Geometry check sheet. Reference: drawing and pictorial views, mm from the part's lowest x, y, z. A direction names the side the tool comes from. Give positions to 0.01 mm unless a question says otherwise; leave off trailing zeros. Loops run counter-clockwise (first coordinate to the right, second up) from the corner with the lowest first, then second, coordinate; pieces in that order, holes last. Notation, with made-up numbers: (20.25, 16.25) -> (68.25, 16.25) arc R24 ccw to (68.25, 34.25) -> close; hole circle Ø1 at (11.5, 43.25). An arc over 180 degrees is marked (long way). Answer in a Markdown table with one row per item. Add a question column.
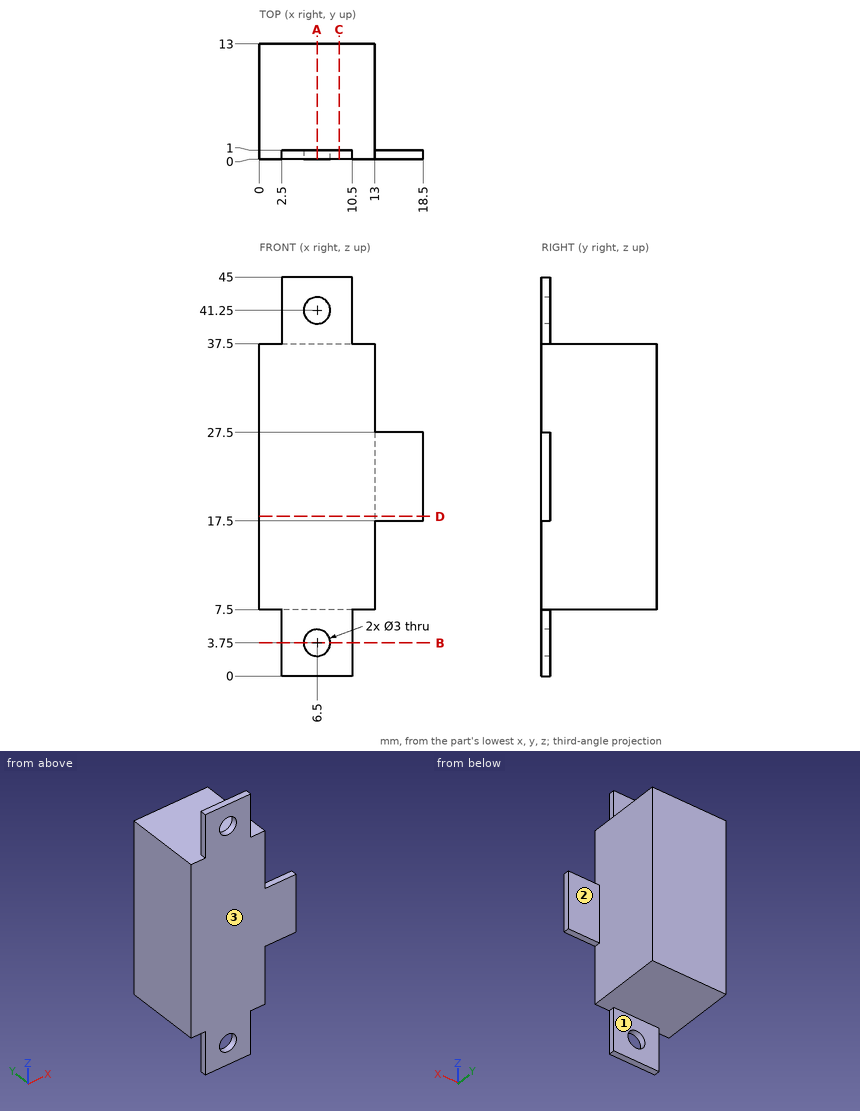
1. Sectioned sample at D-D (z = 18). Enter the section's corners in (x, y), plus the area to 4 significant figures.
2. Material ranges on L1, parallel to Z at x = 6.5, y = 0.6; L2, parallel to Y at x = 14.5, z = 20; L3, parallel to Z at x = 5, y = 10.75, recorded low to high. Write a range as from..to.
3. Gauge pin test, flat ends, axial feed: pin 1 Ø0.8 at (x, y) = (17, 0.5) entering from +Z; pin 2 Ø0.8 at (y, z) = (0.5, 3) entering from +X; pin 3 Ø1.5 at (x, y) = (7, 3) entering from +Z. Record the tip position at first contact, or that the pin passes through.
4. Sectioned sample at C-C (x = 9). Enter the section's corners in (y, z), plus the area to 3 significant figures.
5. Access from +Z, -Z, +X, -X, +Y, -Y to the whole of each face (thin tool, end or side, straight path). Record for the marked faces 1, 2 and 3.
6. Sectioned sample at B-B (z = 3.75). Enter the section's corners in (x, y), plus the area to 3 significant figures.
7. Sectioned sample at A-A (x = 6.5). Enter the section's corners in (y, z), plus the area to 3 significant figures.
Response:
| question | item | result |
|---|---|---|
| 1 | outline | (0, 0) -> (18.5, 0) -> (18.5, 1) -> (13, 1) -> (13, 13) -> (0, 13) -> close |
| 1 | area | 174.5 mm2 |
| 2 | L1 | z = 0..2.25, 5.25..39.75, 42.75..45 |
| 2 | L2 | y = 0..1 |
| 2 | L3 | z = 7.5..37.5 |
| 3 | pin 1 | stops at z = 27.5 |
| 3 | pin 2 | stops at x = 10.5 |
| 3 | pin 3 | stops at z = 37.5 |
| 4 | outline | (0, 0) -> (1, 0) -> (1, 7.5) -> (13, 7.5) -> (13, 37.5) -> (1, 37.5) -> (1, 45) -> (0, 45) -> close |
| 4 | area | 405 mm2 |
| 5 | face 1 | -Z, +X, -X, +Y |
| 5 | face 2 | +Z, -Z, +X, +Y |
| 5 | face 3 | +Z, -Z, +X, -X, -Y |
| 6 | outline | (2.5, 0) -> (5, 0) -> (5, 1) -> (2.5, 1) -> close; (8, 0) -> (10.5, 0) -> (10.5, 1) -> (8, 1) -> close |
| 6 | area | 5.00 mm2 |
| 7 | outline | (0, 0) -> (1, 0) -> (1, 2.25) -> (0, 2.25) -> close; (0, 5.25) -> (1, 5.25) -> (1, 7.5) -> (13, 7.5) -> (13, 37.5) -> (1, 37.5) -> (1, 39.75) -> (0, 39.75) -> close; (0, 42.75) -> (1, 42.75) -> (1, 45) -> (0, 45) -> close |
| 7 | area | 399 mm2 |
